Read the model definition and answer for the solid it produces. Units are mm, in the model's axes. Coordinates: 2 decimals unless noted, no trailing zeros. Loops run counter-clockwise (first coordinate to the right, second up) from the corner with the lowest first, then second, coordinate; pieces in that order, holes last.
Q1. Section A-A (y = -65) is taken. Give the vertices of the cut face in (x, z) (3 decimals), then the cut area to 3 significant figures.
Q2. Section B-B (z = 1.85) is taken. Count the separate pieces of the cut face and the enclosed holes in it, then the cut area to 3 significant figures.
Q3. Flat-ended cylindrical pins translate along their axes: P1, Ø8, axis at x = 240, y = 81.5, coming from the -Z side; P2, Ø1, axis at x = 291, z = 2, coming from the +Y side (3 decimals); P3, Ø1.6, axis at y = -47, z = 1.5, coming from the +X side; P4, Ø1, axis at y = -51, z = 2, coming from the -X side. Find the tip coordinate at first contact, or state that the pin passes through.
Q4. Section D-D (x = 251.5) is taken. Give the vertices of the cut face in (y, z) (3 decimals).
Q5. Straight lines are drawn through the part: line 1 (Y direction, x = -21, z = 0.3); line 2 (X direction, y = -76.5, z = 0.95); line 3 (Y direction, x = 117.5, z = 2.95). For each, find the intervals that lie inside material, in ascending order.
from build123d import *

# Parameters (mm, degrees)
F0_W     = 76.2
F0_H     = 12.7
F1_DEPTH = 3.175
F2_DEPTH = 12.7


# Not quite as in the source:
# - a length typed as a fraction of an inch, garbled in the dataset ("3 / 203.2 mm" for 3/8 in), is restored


with BuildPart() as f1:
    # F0 (on Top) → F1 (new body)
    with BuildSketch(Plane.XY):
        Polygon((285.7501016, -19.0500762), (304.8001016, -19.0500762), (304.8001016, 53.9749238), (222.2501016, 104.7749238), (-222.2500762, 104.7749238), (-304.8000762, 53.9749238), (-304.8000762, -19.0500762), (-285.7500762, -19.0500762), (-285.7500762, -73.0248984), (-304.8000762, -73.0248984), (-304.8000762, -104.7748984), (-109.5373984, -104.7748984), (-109.5373984, -67.4683182), (-244.475254, -67.4683182), (-244.475254, -46.8308182), (-162.5825794541, -46.8308182), (-196.8829692, -12.5304042), (-194.6378124, -10.285222), (-158.7168276, -46.2063846), (-159.3413106539, -46.8308182), (-137.1825794541, -46.8308182), (-171.4829692, -12.5304042), (-169.2378124, -10.285222), (-133.3168276, -46.2063846), (-133.9413106539, -46.8308182), (-111.7825794541, -46.8308182), (-146.0829692, -12.5304042), (-143.8378124, -10.285222), (-107.9168276, -46.2063846), (-108.5413106539, -46.8308182), (-86.3825794541, -46.8308182), (-120.6829692, -12.5304042), (-118.4378124, -10.285222), (-82.5168276, -46.2063846), (-83.1413106539, -46.8308182), (-60.9824096755, -46.8308182), (-95.2829692, -12.5304042), (-93.0378124, -10.285222), (-57.1170054, -46.2063846), (-57.7413895461, -46.8308182), (-35.5824096755, -46.8308182), (-69.8829692, -12.5304042), (-67.6378124, -10.285222), (-31.7170054, -46.2063846), (-32.3413895461, -46.8308182), (-10.1824176969, -46.8308182), (-44.483147, -12.5304042), (-42.2376346, -10.285222), (-6.3170054, -46.2063846), (-6.9413895461, -46.8308182), (11.3860423894, -46.8308182), (10.7618784, -46.2065624), (46.682533, -10.2855776), (48.9280454, -12.5307598), (14.6276231923, -46.8308182), (36.7860423894, -46.8308182), (36.1618784, -46.2065624), (72.082533, -10.2855776), (74.3280454, -12.5307598), (40.0276231923, -46.8308182), (62.1860423894, -46.8308182), (61.5618784, -46.2065624), (97.482533, -10.2855776), (99.7280454, -12.5307598), (65.4276231923, -46.8308182), (87.5860423894, -46.8308182), (86.9618784, -46.2065624), (122.882533, -10.2855776), (125.1280454, -12.5307598), (90.8276231923, -46.8308182), (112.9860423894, -46.8308182), (112.3618784, -46.2065624), (148.282533, -10.2855776), (150.5280454, -12.5307598), (116.2276231923, -46.8308182), (138.3860423894, -46.8308182), (137.7618784, -46.2065624), (173.682533, -10.2855776), (175.9280454, -12.5307598), (141.6276231923, -46.8308182), (163.7860423894, -46.8308182), (163.1618784, -46.2065624), (199.082533, -10.2855776), (201.3280454, -12.5307598), (167.0276231923, -46.8308182), (244.474746, -46.8308182), (244.474746, -67.4683182), (109.5376016, -67.4683182), (109.5376016, -104.7748984), (304.8001016, -104.7748984), (304.8001016, -73.0248984), (285.7501016, -73.0248984), align=None)
        with Locations((-165.052883, -79.3748984)):
            Rectangle(F0_W, F0_H, mode=Mode.SUBTRACT)
        with Locations((165.1001016, -79.3748984)):
            Rectangle(F0_W, F0_H, mode=Mode.SUBTRACT)
        Polygon((-158.7168276, 33.506918), (-194.6378124, -2.4142192), (-196.8829692, -0.1690624), (-160.9620098, 35.7519224), align=None, mode=Mode.SUBTRACT)
        Polygon((-133.3168276, 33.506918), (-169.2378124, -2.4142192), (-171.4829692, -0.1690624), (-135.5620098, 35.7519224), align=None, mode=Mode.SUBTRACT)
        Polygon((-107.9168276, 33.506918), (-143.8378124, -2.4142192), (-146.0829692, -0.1690624), (-110.1620098, 35.7519224), align=None, mode=Mode.SUBTRACT)
        Polygon((-82.5168276, 33.506918), (-118.4378124, -2.4142192), (-120.6829692, -0.1690624), (-84.7620098, 35.7519224), align=None, mode=Mode.SUBTRACT)
        Polygon((-57.1170054, 33.506918), (-93.0378124, -2.4142192), (-95.2829692, -0.1690624), (-59.361832, 35.7519224), align=None, mode=Mode.SUBTRACT)
        Polygon((-31.7170054, 33.506918), (-67.6378124, -2.4142192), (-69.8829692, -0.1690624), (-33.961832, 35.7519224), align=None, mode=Mode.SUBTRACT)
        Polygon((-6.3170054, 33.506918), (-42.2376346, -2.4142192), (-44.483147, -0.1690624), (-8.561832, 35.7519224), align=None, mode=Mode.SUBTRACT)
        Polygon((13.006705, 35.752278), (48.9280454, -0.1687068), (46.682533, -2.413889), (10.7618784, 33.5070958), align=None, mode=Mode.SUBTRACT)
        Polygon((38.406705, 35.752278), (74.3280454, -0.1687068), (72.082533, -2.413889), (36.1618784, 33.5070958), align=None, mode=Mode.SUBTRACT)
        Polygon((63.806705, 35.752278), (99.7280454, -0.1687068), (97.482533, -2.413889), (61.5618784, 33.5070958), align=None, mode=Mode.SUBTRACT)
        Polygon((89.206705, 35.752278), (125.1280454, -0.1687068), (122.882533, -2.413889), (86.9618784, 33.5070958), align=None, mode=Mode.SUBTRACT)
        Polygon((114.606705, 35.752278), (150.5280454, -0.1687068), (148.282533, -2.413889), (112.3618784, 33.5070958), align=None, mode=Mode.SUBTRACT)
        Polygon((140.006705, 35.752278), (175.9280454, -0.1687068), (173.682533, -2.413889), (137.7618784, 33.5070958), align=None, mode=Mode.SUBTRACT)
        Polygon((165.406705, 35.752278), (201.3280454, -0.1687068), (199.082533, -2.413889), (163.1618784, 33.5070958), align=None, mode=Mode.SUBTRACT)
        Polygon((109.5376016, -50.7998984), (109.5376016, -67.4683182), (244.474746, -67.4683182), (244.474746, -46.8308182), (167.0276231923, -46.8308182), (165.406705, -48.4517192), (163.7860423894, -46.8308182), (141.6276231923, -46.8308182), (140.006705, -48.4517192), (138.3860423894, -46.8308182), (116.2276231923, -46.8308182), (114.606705, -48.4517192), (112.9860423894, -46.8308182), (90.8276231923, -46.8308182), (89.206705, -48.4517192), (87.5860423894, -46.8308182), (65.4276231923, -46.8308182), (63.806705, -48.4517192), (62.1860423894, -46.8308182), (40.0276231923, -46.8308182), (38.406705, -48.4517192), (36.7860423894, -46.8308182), (14.6276231923, -46.8308182), (13.006705, -48.4517192), (11.3860423894, -46.8308182), (-6.9413895461, -46.8308182), (-8.561832, -48.451389), (-10.1824176969, -46.8308182), (-32.3413895461, -46.8308182), (-33.961832, -48.451389), (-35.5824096755, -46.8308182), (-57.7413895461, -46.8308182), (-59.361832, -48.451389), (-60.9824096755, -46.8308182), (-83.1413106539, -46.8308182), (-84.7620098, -48.451389), (-86.3825794541, -46.8308182), (-108.5413106539, -46.8308182), (-110.1620098, -48.451389), (-111.7825794541, -46.8308182), (-133.9413106539, -46.8308182), (-135.5620098, -48.451389), (-137.1825794541, -46.8308182), (-159.3413106539, -46.8308182), (-160.9620098, -48.451389), (-162.5825794541, -46.8308182), (-244.475254, -46.8308182), (-244.475254, -67.4683182), (-109.5373984, -67.4683182), (-109.5373984, -50.7998984), align=None)
    extrude(amount=F1_DEPTH)

    # F2 (cut): faces of the model
    f2_faces = [f1.faces().sort_by_distance(p)[0] for p in [
        (-207.1687373, -104.7748984, 1.5875),
        (207.1688516, -104.7748984, 1.5875),
    ]]
    extrude(f2_faces, amount=-F2_DEPTH, mode=Mode.SUBTRACT)


solid = f1.part
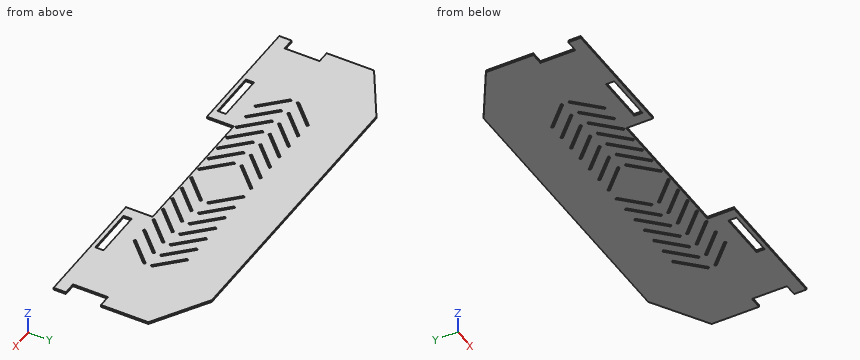
Numbers:
1. outline: (-285.75, 0) - (-109.537, 0) - (-109.537, 3.175) - (-285.75, 3.175) - close; (109.538, 0) - (285.75, 0) - (285.75, 3.175) - (109.538, 3.175) - close
1. area: 1,120 mm2
2. separate pieces: 1
2. enclosed holes: 30
2. area: 98,300 mm2
3. P1: stops at z = 0
3. P2: stops at y = 62.775
3. P3: stops at x = 285.75
3. P4: stops at x = -285.75
4. outline: (-92.075, 0) - (86.775, 0) - (86.775, 3.175) - (-92.075, 3.175) - close
5. line 1: y = -50.8 to -36.01, -31.52 to 18.82, 23.31 to 104.77
5. line 2: x = -304.8 to -203.15, -126.95 to -109.54, 109.54 to 127, 203.2 to 304.8
5. line 3: y = -92.07 to -45.56, -41.07 to -20.16, -15.67 to 2.97, 7.46 to 28.37, 32.86 to 104.77
